Autodesk Inventor part; units mm, degrees
ref_plane "YZ Plane" through (0, 0, 0) normal (1, 0, 0) x (0, 1, 0)
ref_plane "XZ Plane" through (0, 0, 0) normal (0, 1, 0) x (-1, 0, 0)
ref_plane "XY Plane" through (0, 0, 0) normal (0, 0, 1) x (1, 0, 0)
sketch "草圖1" plane through (0, 0, 0) normal (0, 1, 0) x (-1, 0, 0)
  line L0 (2.5, 2.5) -> (-2.5, 2.5)
  line L1 (-2.5, 2.5) -> (-2.5, -2.5)
  line L2 (-2.5, -2.5) -> (2.5, -2.5)
  line L3 (2.5, -2.5) -> (2.5, 2.5)
  circle A0 centre (0, 0) radius 1.7
  point P0 (2.5, 0)
  point P1 (0, -2.5)
  dimension "d0" = 5
  dimension "d1" = 5
  dimension "d2" = 3.4
extrude "擠出1" add sketch "草圖1" along normal blind 6 contours L3 L2 L1 L0 | A0
extrude "擠出2" cut sketch "草圖1" along normal blind 1.5 contours A0
sketch "草圖2" plane through (0, 6, 0) normal (0, 1, 0) x (1, 0, 0)
  line L0 (2.5, -2.5) -> (2.5, 2.5)
  line L1 (2.5, 2.5) -> (-2.5, 2.5)
  line L2 (-2.5, 2.5) -> (-2.5, -2.5)
  line L3 (-2.5, -2.5) -> (2.5, -2.5)
  point P0 (0, 0)
extrude "擠出3" add sketch "草圖2" along normal blind 15 draft -30
sketch "草圖3" plane through (2.5, 0, -2.5) normal (0, 0, -1) x (-1, 0, 0)
  line L0 (0, 0) -> (5, 0)
  line L1 (5, 0) -> (5, 6)
  line L2 (0, 6) -> (5, 6)
  line L3 (0, 0) -> (0, 6)
  line L4 (3, 4) -> (3, 2)
  line L5 (3, 2) -> (2, 2)
  line L6 (2, 2) -> (2, 4)
  line L7 (2, 4) -> (3, 4)
  point P0 (2.5, 0)
  dimension "d9" = 2
extrude "擠出4" add sketch "草圖3" along normal blind 2.5 contours L4 L5 L6 L7
mirror "鏡射1" about plane through (0, 0, 0) normal (0, 0, 1) of "擠出4"
properties part number "110033226_ipt_21_柵欄"
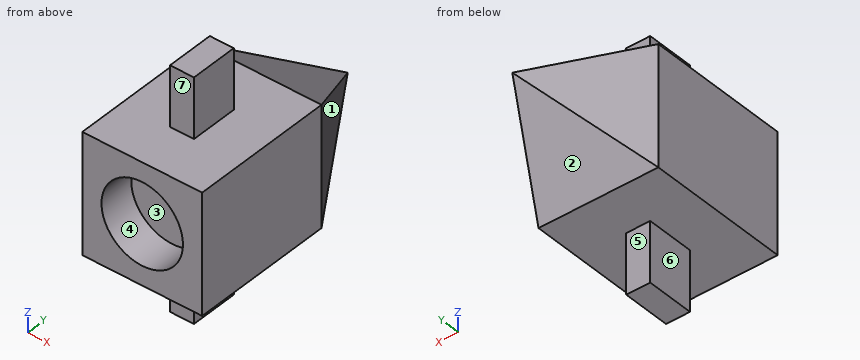
Read the model definition and answer for the solid it produces. Units are mm, in the model's axes. Face numbers are marked on the shaded views. A direction names the side the tool comes from. Give positions to 0.01 mm unless a question says otherwise; leave off trailing zeros. Loops run counter-clockwise (first coordinate to the right, second up) from the corner with the lowest first, then second, coordinate; pieces in that order, holes last.
Item 1: The part is cut by section D-D (z = -4). Write down the section's boundary in (x, y).
Item 2: The part is cut by section C-C (x = -1.1). Write down the section's boundary in (y, z).
Item 3: The part is cut by section A-A (y = 3). Write down the section's boundary in (x, z), and give its area (3 significant figures).
Item 4: The part is cut by section B-B (z = 1). Write down the section's boundary in (x, y).
Item 5: Each of these flat-tipped pins is pushed along its axis until it touches: pin 1 Ø0.5 at (x, z) = (0, 4.5) entering from -Y; pin 2 Ø1 at (y, z) = (3, 4) entering from +X; pin 3 Ø2 at (x, z) = (-1.5, 0) entering from -Y; pin 4 Ø2 at (x, z) = (0, -3) entering from +Y. Where does it stop, or does it pass through?
Item 6: Find the intervals of material crossed by line 1 along Z through (x, y) = (0, 1.2); line 2 along Z through (x, y) = (1.1, 1.75); line 3 along X through (y, z) = (3.25, 4), in increasing order.
Item 7: For the marked faces 4, 5, 6 and 7, determine the directions among +Z, -Z, +X, -X, +Y, -Y from which every point of the face is accessible in a straight line to the end or side of a thin tool.
Item 8: The mould has two halves that part along Z. Classify the marked faces 1, 2 and 3: released by +Z, released by -Z, zero draft, split by the parting line, or undercut.
Taken from the geometry:
1. outline: (-0.5, 2) - (0.5, 2) - (0.5, 4) - (-0.5, 4) - close
2. outline: (0, -2.5) - (6, -2.5) - (8.42, -1.1) - (8.42, 1.1) - (6, 2.5) - (0, 2.5) - (0, 1.3) - (1.5, 1.3) - (1.5, -1.3) - (0, -1.3) - close
3. outline: (-2.5, -2.5) - (-0.5, -2.5) - (-0.5, -5) - (0.5, -5) - (0.5, -2.5) - (2.5, -2.5) - (2.5, 2.5) - (0.5, 2.5) - (0.5, 5) - (-0.5, 5) - (-0.5, 2.5) - (-2.5, 2.5) - close
3. area: 30.0 mm2
4. outline: (-2.5, 0) - (-1.37, 0) - (-1.37, 1.5) - (1.37, 1.5) - (1.37, 0) - (2.5, 0) - (2.5, 6) - (1, 8.6) - (-1, 8.6) - (-2.5, 6) - close
5. pin 1: stops at y = 2
5. pin 2: stops at x = 0.5
5. pin 3: stops at y = 0
5. pin 4: stops at y = 6.87
6. line 1: z = -2.5 to -1.7, 1.7 to 2.5
6. line 2: z = -2.5 to 2.5
6. line 3: x = -0.5 to 0.5
7. face 4: -Y
7. face 5: -Z, +X, -X, +Y
7. face 6: -Z, -X, +Y, -Y
7. face 7: +Z, +X, -X, -Y
8. face 1: zero draft
8. face 2: released by -Z
8. face 3: undercut
